```python
from build123d import *

# Parameters (mm, degrees)
SKETCH1_R           = 2
BOSS_EXTRUDE1_DEPTH = 21.75
CHAMFER1_SIZE       = 0.25
SKETCH2_OUTSIDE_W   = 10.494
SKETCH2_OUTSIDE_H   = 10.494
CUT_EXTRUDE1_DEPTH  = 12


with BuildPart() as part:
    # Sketch1 → Boss-Extrude1 (new body)
    with BuildSketch(Plane(origin=(0, 0, 0), x_dir=(1, 0, 0), z_dir=(0, 1, 0))):
        with Locations(Location((0, 0, 0), (0, 0, 270))):
            Circle(SKETCH1_R)
    extrude(amount=BOSS_EXTRUDE1_DEPTH)

    # Chamfer1
    chamfer1_edges = [part.edges().sort_by_distance(p)[0] for p in [
        (0, 21.75, -2),
    ]]
    chamfer(chamfer1_edges, length=CHAMFER1_SIZE)

    # Sketch2 outside → Cut-Extrude1 (cut)
    with BuildSketch(Plane(origin=(0, 21.75, 0), x_dir=(1, 0, 0), z_dir=(0, 1, 0))):
        Rectangle(SKETCH2_OUTSIDE_W, SKETCH2_OUTSIDE_H)
        with BuildLine():
            Line((-1.4, 1.428285686), (-1.4, -1.428285686))
            ThreePointArc((-1.4, -1.428285686), (2, 0), (-1.4, 1.428285686))
        make_face(mode=Mode.SUBTRACT)
    extrude(amount=-CUT_EXTRUDE1_DEPTH, mode=Mode.SUBTRACT)


solid = part.part
```
The listing builds one solid part. Answer for the finished solid, in the listing's coordinates (mm). A direction names the side the tool comes from. Give positions to 0.01 mm unless a question says otherwise; leave off trailing zeros. Order: outer loops, then holes, each group sorted by start corner. A loop starts at its lowest first (then second) coordinate and runs counter-clockwise, first axis right, second up. Notation, with made-up numbers: M 63,32 L 91,32 A25 cw 91,53 Z; hole C 38.25,-2.5 d2. An arc over 180 degrees is marked long. Put each result on its own line as item: value. Start each with the question number.
Item 1: Which of the six approach directions +Z, -Z, +X, -X, +Y, -Y give full straight-line access (tool end or side, diameter ignored) to faces 1 (the face through (0, 21.75, 0)), 2 (the face through (-1.4, 16, 0))?
Item 2: The part is cut by section A-A, the plane z = 0. Determine the outline of the cut face in (x, y), and give its area (3 significant figures).
Item 3: The part is cut by section C-C, the plane y = 3.75. Determine the outline of the cut face in (x, z).
Item 4: The part is cut by section B-B, the plane y = 17.5. Determine the outline of the cut face in (x, z).
Item 5: Find the intervals of material crossed by line 1 along Y through (x, z) = (-1.55, -0.1); line 2 along Z through (x, y) = (0.3, 1.25); line 3 along Z through (x, y) = (1.3, 5.75), in increasing order.
Item 6: A flat-ended cylindrical pin translates along its axis: P1, Ø1.5, axis at y = 14, z = 0, coming from the -X side. Find the tip coordinate at first contact, or state that the pin passes through.
Answer key:
1. face 1: +Z, -Z, +X, -X, +Y
1. face 2: +Z, -Z, -X, +Y
2. outline: M -2,0 L 2,0 L 2,21.5 L 1.75,21.75 L -1.4,21.75 L -1.4,9.75 L -2,9.75 Z
2. area: 79.8 mm²
3. outline: C 0,0 d4
4. outline: M -1.4,-1.43 A2 ccw long -1.4,1.43 Z
5. line 1: y = 0 to 9.75
5. line 2: z = -1.98 to 1.98
5. line 3: z = -1.52 to 1.52
6. P1: stops at x = -1.4
